For this review, take the finished solid that the model builds, in its own axes (mm). A direction names the side the tool comes from. Give positions to 0.01 mm unless a question says otherwise; leave off trailing zeros. Loops run counter-clockwise (first coordinate to the right, second up) from the corner with the lowest first, then second, coordinate; pieces in that order, holes last. Notation, with made-up numbers: M 34.5,-23 L 86.5,-23 A9 ccw 86.5,-14 Z; hole C 73,20 d2. An arc over 180 degrees is marked long. Use CSV: the item, a comma, the result in double quotes. Start each with the question number.
1. Take a section at A-A, the plane x = 0. Write out the cut boundary in (y, z).
2. Take a section at C-C, the plane y = -0.45. Write out the cut boundary in (x, z).
3. The part is to be moulded in two halves that separate along Z. For faces 3 (the face through (-0.17, -0.79, 25.26)), 4 (the face through (0, 0, 1)), 5 (the face through (0, -1, 36.703)), 6 (the face through (-0.1, -0.8, -20.7)), say which applies: pulls with the +Z half, pulls with the -Z half, needs draft (parallel to the pull), parting line crosses it, or undercut.
4. Take a section at B-B, the plane z = -23.5. Write out the cut boundary in (x, y), and give its area (3 significant figures).
5. Tool access review of faces 1 (the face through (19.05, -1, -1)), 2 (the face through (-5.207, -1, -31)): name each direction out of +Z, -Z, +X, -X, +Y, -Y from which nothing blocks a thin tool from reaching the whole face with its end or side.
6. To check wall thickness, follow line 1 (Z direction, x = 0, y = -0.95); line 2 (X direction, y = -1.3, z = -24); line 3 (Z direction, x = 1, y = -1.1). State the ranges of each line that lie inside material, in increasing order. Write a range as [from, to].
from build123d import *

# Parameters (mm, degrees)
F0_R     = 1.27
F1_DEPTH = 1.6002


with BuildPart() as f1:
    # F0 (on Front) → F1 (new body)
    with BuildSketch(Plane.XZ):
        with BuildLine():
            Line((5.207, -36.703), (19.05, -36.703))
            Line((19.05, -36.703), (19.05, 36.703))
            Line((19.05, 36.703), (-19.05, 36.703))
            Line((-19.05, 36.703), (-19.05, -36.703))
            Line((-19.05, -36.703), (-5.207, -36.703))
            Line((-5.207, -36.703), (-5.207, -25.908))
            ThreePointArc((-5.207, -25.908), (0, -20.701), (5.207, -25.908))
            Line((5.207, -25.908), (5.207, -36.703))
        make_face()
        with Locations((0, 24.003)):
            Circle(F0_R, mode=Mode.SUBTRACT)
    extrude(amount=F1_DEPTH)


solid = f1.part
Result set:
1,outline,"M -1.6,-20.7 L 0,-20.7 L 0,22.73 L -1.6,22.73 Z; M -1.6,25.27 L 0,25.27 L 0,36.7 L -1.6,36.7 Z"
2,outline,"M -19.05,-36.7 L -5.21,-36.7 L -5.21,-25.91 A5.21 cw 5.21,-25.91 L 5.21,-36.7 L 19.05,-36.7 L 19.05,36.7 L -19.05,36.7 Z; hole C 0,24 d2.54"
3,face 3,"undercut"
3,face 4,"needs draft"
3,face 5,"pulls with the +Z half"
3,face 6,"pulls with the -Z half"
4,outline,"M -19.05,-1.6 L -4.62,-1.6 L -4.62,0 L -19.05,0 Z; M 4.62,-1.6 L 19.05,-1.6 L 19.05,0 L 4.62,0 Z"
4,area,"46.2 mm2"
5,face 1,"+Z, -Z, +X, +Y, -Y"
5,face 2,"-Z, +Y, -Y"
6,line 1,"[-20.7, 22.73], [25.27, 36.7]"
6,line 2,"[-19.05, -4.84], [4.84, 19.05]"
6,line 3,"[-20.8, 23.22], [24.79, 36.7]"
